```python
from build123d import *

# Parameters (mm, degrees)
F0_W      = 130
F0_H      = 75
F1_DEPTH  = 12
F3_DEPTH  = 319
F5_DEPTH  = 100
F6_W      = 220
F6_H      = 75
F7_DEPTH  = 12
F9_D      = 12
F9_DEPTH  = 12
F9_TIP    = 3.6051637142
F11_D     = 12
F11_DEPTH = 12
F11_TIP   = 3.6051637142


# Not quite as in the source:
# - a feature names something its author has since deleted; it is built from what else it names


with BuildPart() as f1:
    # F0 (on Top) → F1 (new body)
    with BuildSketch(Plane.XY):
        with Locations((65, -37.5)):
            Rectangle(F0_W, F0_H)
    extrude(amount=F1_DEPTH)

    # F2 (on face) → F3 (join)
    with BuildSketch(Plane.XY.offset(12)):
        with BuildLine():
            ThreePointArc((90.4, -18.45), (88.5401280605, -13.9598719395), (84.05, -12.1))
            Line((84.05, -12.1), (45.95, -12.1))
            ThreePointArc((45.95, -12.1), (41.4598719395, -13.9598719395), (39.6, -18.45))
            Line((39.6, -18.45), (39.6, -56.55))
            ThreePointArc((39.6, -56.55), (41.4598719395, -61.0401280605), (45.95, -62.9))
            Line((45.95, -62.9), (84.05, -62.9))
            ThreePointArc((84.05, -62.9), (88.5401280605, -61.0401280605), (90.4, -56.55))
            Line((90.4, -56.55), (90.4, -18.45))
        make_face()
        with BuildLine():
            Line((52.3, -18.45), (77.7, -18.45))
            ThreePointArc((77.7, -18.45), (82.1901280605, -20.3098719395), (84.05, -24.8))
            Line((84.05, -24.8), (84.05, -50.2))
            ThreePointArc((84.05, -50.2), (82.1901280605, -54.6901280605), (77.7, -56.55))
            Line((77.7, -56.55), (52.3, -56.55))
            ThreePointArc((52.3, -56.55), (47.8098719395, -54.6901280605), (45.95, -50.2))
            Line((45.95, -50.2), (45.95, -24.8))
            ThreePointArc((45.95, -24.8), (47.8098719395, -20.3098719395), (52.3, -18.45))
        make_face(mode=Mode.SUBTRACT)
    extrude(amount=F3_DEPTH)

    # F4 (on face) → F5 (cut)
    with BuildSketch(Plane.YZ.offset(90.4)):
        Polygon((-62.9, 305), (-12.1, 331), (-62.9, 331), align=None)
    extrude(amount=-F5_DEPTH, mode=Mode.SUBTRACT)

    # F6 (on face) → F7 (join)
    with BuildSketch(Plane(origin=(0, -136.7557973863, 267.1997887393), x_dir=(1, 0, 0), z_dir=(0, -0.4556049895, 0.8901820564))):
        with Locations((65, 111.5005595453)):
            Rectangle(F6_W, F6_H)
        with BuildLine():
            Line((90.4, 132.9006763674), (90.4, 90.1004427232))
            add(Edge.make_bspline(
                [(90.4, 90.1004427232), (90.4, 82.9670704491), (84.05, 82.9670704491)],
                knots=[4.7123889804, 4.7123889804, 4.7123889804, 6.2831853072, 6.2831853072, 6.2831853072], degree=2, weights=[1, 0.7071067812, 1]))
            Line((84.05, 82.9670704491), (45.95, 82.9670704491))
            add(Edge.make_bspline(
                [(45.95, 82.9670704491), (39.6, 82.9670704491), (39.6, 90.1004427232)],
                knots=[0, 0, 0, 1.5707963268, 1.5707963268, 1.5707963268], degree=2, weights=[1, 0.7071067812, 1]))
            Line((39.6, 90.1004427232), (39.6, 132.9006763674))
            add(Edge.make_bspline(
                [(39.6, 132.9006763674), (39.6, 140.0340486414), (45.95, 140.0340486414)],
                knots=[1.5707963268, 1.5707963268, 1.5707963268, 3.1415926536, 3.1415926536, 3.1415926536], degree=2, weights=[1, 0.7071067812, 1]))
            Line((45.95, 140.0340486414), (84.05, 140.0340486414))
            add(Edge.make_bspline(
                [(84.05, 140.0340486414), (90.4, 140.0340486414), (90.4, 132.9006763674)],
                knots=[3.1415926536, 3.1415926536, 3.1415926536, 4.7123889804, 4.7123889804, 4.7123889804], degree=2, weights=[1, 0.7071067812, 1]))
        make_face(mode=Mode.SUBTRACT)
        with BuildLine():
            add(Edge.make_bspline(
                [(90.4, 90.1004427232), (90.4, 82.9670704491), (84.05, 82.9670704491)],
                knots=[4.7123889804, 4.7123889804, 4.7123889804, 6.2831853072, 6.2831853072, 6.2831853072], degree=2, weights=[1, 0.7071067812, 1]))
            Line((90.4, 90.1004427232), (90.4, 132.9006763674))
            add(Edge.make_bspline(
                [(84.05, 140.0340486414), (90.4, 140.0340486414), (90.4, 132.9006763674)],
                knots=[3.1415926536, 3.1415926536, 3.1415926536, 4.7123889804, 4.7123889804, 4.7123889804], degree=2, weights=[1, 0.7071067812, 1]))
            Line((84.05, 140.0340486414), (45.95, 140.0340486414))
            add(Edge.make_bspline(
                [(39.6, 132.9006763674), (39.6, 140.0340486414), (45.95, 140.0340486414)],
                knots=[1.5707963268, 1.5707963268, 1.5707963268, 3.1415926536, 3.1415926536, 3.1415926536], degree=2, weights=[1, 0.7071067812, 1]))
            Line((39.6, 132.9006763674), (39.6, 90.1004427232))
            add(Edge.make_bspline(
                [(45.95, 82.9670704491), (39.6, 82.9670704491), (39.6, 90.1004427232)],
                knots=[0, 0, 0, 1.5707963268, 1.5707963268, 1.5707963268], degree=2, weights=[1, 0.7071067812, 1]))
            Line((45.95, 82.9670704491), (84.05, 82.9670704491))
        make_face()
        with BuildLine():
            Line((52.3, 132.9006763674), (77.7, 132.9006763674))
            add(Edge.make_bspline(
                [(77.7, 132.9006763674), (84.05, 132.9006763674), (84.05, 125.7673040934)],
                knots=[3.1415926536, 3.1415926536, 3.1415926536, 4.7123889804, 4.7123889804, 4.7123889804], degree=2, weights=[1, 0.7071067812, 1]))
            Line((84.05, 125.7673040934), (84.05, 97.2338149972))
            add(Edge.make_bspline(
                [(84.05, 97.2338149972), (84.05, 90.1004427232), (77.7, 90.1004427232)],
                knots=[4.7123889804, 4.7123889804, 4.7123889804, 6.2831853072, 6.2831853072, 6.2831853072], degree=2, weights=[1, 0.7071067812, 1]))
            Line((77.7, 90.1004427232), (52.3, 90.1004427232))
            add(Edge.make_bspline(
                [(52.3, 90.1004427232), (45.95, 90.1004427232), (45.95, 97.2338149972)],
                knots=[0, 0, 0, 1.5707963268, 1.5707963268, 1.5707963268], degree=2, weights=[1, 0.7071067812, 1]))
            Line((45.95, 97.2338149972), (45.95, 125.7673040934))
            add(Edge.make_bspline(
                [(45.95, 125.7673040934), (45.95, 132.9006763674), (52.3, 132.9006763674)],
                knots=[1.5707963268, 1.5707963268, 1.5707963268, 3.1415926536, 3.1415926536, 3.1415926536], degree=2, weights=[1, 0.7071067812, 1]))
        make_face(mode=Mode.SUBTRACT)
        with BuildLine():
            add(Edge.make_bspline(
                [(77.7, 132.9006763674), (84.05, 132.9006763674), (84.05, 125.7673040934)],
                knots=[3.1415926536, 3.1415926536, 3.1415926536, 4.7123889804, 4.7123889804, 4.7123889804], degree=2, weights=[1, 0.7071067812, 1]))
            Line((77.7, 132.9006763674), (52.3, 132.9006763674))
            add(Edge.make_bspline(
                [(45.95, 125.7673040934), (45.95, 132.9006763674), (52.3, 132.9006763674)],
                knots=[1.5707963268, 1.5707963268, 1.5707963268, 3.1415926536, 3.1415926536, 3.1415926536], degree=2, weights=[1, 0.7071067812, 1]))
            Line((45.95, 125.7673040934), (45.95, 97.2338149972))
            add(Edge.make_bspline(
                [(52.3, 90.1004427232), (45.95, 90.1004427232), (45.95, 97.2338149972)],
                knots=[0, 0, 0, 1.5707963268, 1.5707963268, 1.5707963268], degree=2, weights=[1, 0.7071067812, 1]))
            Line((52.3, 90.1004427232), (77.7, 90.1004427232))
            add(Edge.make_bspline(
                [(84.05, 97.2338149972), (84.05, 90.1004427232), (77.7, 90.1004427232)],
                knots=[4.7123889804, 4.7123889804, 4.7123889804, 6.2831853072, 6.2831853072, 6.2831853072], degree=2, weights=[1, 0.7071067812, 1]))
            Line((84.05, 97.2338149972), (84.05, 125.7673040934))
        make_face()
    extrude(amount=F7_DEPTH)

    # F9
    with Locations(Plane(origin=(0, -142.2230572602, 277.8819734162), x_dir=(1, 0, 0), z_dir=(0, -0.4556049895, 0.8901820564))):
        with Locations((-30, 89.0005595453), (100, 89.0005595453), (160, 89.0005595453), (160, 119.0005595453), (100, 119.0005595453), (30, 119.0005595453), (-30, 119.0005595453), (30, 89.0005595453)):
            Hole(F9_D / 2, depth=F9_DEPTH)
            with Locations((0, 0, -(F9_DEPTH + F9_TIP / 2))):  # 118° drill point
                Cone(0, F9_D / 2, F9_TIP, mode=Mode.SUBTRACT)

    # F11 (one way)
    with BuildSketch(Plane.XY.offset(12)):
        with Locations((15, -15), (15, -60), (115, -60), (115, -15)):
            Circle(F11_D / 2)
    extrude(amount=-F11_DEPTH, mode=Mode.SUBTRACT)
    with Locations(Plane.XY.offset(12)):
        with Locations((15, -15), (15, -60), (115, -60), (115, -15)):
            with Locations((0, 0, -(F11_DEPTH + F11_TIP / 2))):  # 118° drill point
                Cone(0, F11_D / 2, F11_TIP, mode=Mode.SUBTRACT)


solid = f1.part
```
Source: CAD feature listing. Evaluate the final solid. Frame: model axes, mm. A direction names the side the tool comes from. Give positions to 0.01 mm unless a question says otherwise; leave off trailing zeros. Write each loop counter-clockwise with the first axis right and the second up, starting at its lowest first coordinate (ties: lowest second). Pieces come first, ordered by that corner, then holes.
1. Pull-direction query (X, two-part tool) for faces 1 (the face through (84.05, -37, 166)), 2 (the face through (88.59, -14.01, 169.27)), 3 (the face through (93, -37, 12)); classes: +X half, -X half, draft (parallel to the pull), parting line (faces both ways), or undercut.
2. First-contact query: pin 1 (11.5 mm diameter, centred on x = 57, z = 125, fed in from +Y); pin 2 (12.5 mm diameter, centred on y = -36.5, z = 126.5, fed in from +X); pin 3 (2 mm diameter, centred on y = -34, z = 204, fed in from -X). Flat tips, straight axial feed; report the tip coordinate or a pass-through.
3. Access query for faces 4 (the face through (64.73, -37.23, 318.14)), 5 (the face through (65, -12.1, 169)), 6 (the face through (64, -37, 0)), 7 (the face through (63.46, -73.577, 306.181)), 8 (the face through (20.54, -62.3, 6.08)). Directions: +Z, -Z, +X, -X, +Y, -Y. A direction counts if a zero-diameter tool reaches every point of the face in a straight line with its end or side. Return the directions, or none.
4. Section query A-A (x = 15). Return the cut outline in (y, z).
5. Section query C-C (x = 59). Return the cut outline in (y, z).
6. Section query D-D (x = 115.5). Return the cut outline in (y, z), then the cut area to 3 significant figures.
7. Material intervals for line 1 along Y through (x, z) = (15, 6); line 2 along X through (y, z) = (-28, 307); line 3 along Z through (x, y) = (112, -39), sorted ascending.
8. Section query B-B (z = 151.5). Return the cut outline in (x, y), then the cut area to 3 significant figures.
Output values:
1. face 1: undercut
1. face 2: +X half
1. face 3: draft
2. pin 1: stops at y = -12.1
2. pin 2: stops at x = 90.4
2. pin 3: stops at x = 39.6
3. face 4: none
3. face 5: +X, -X, +Y
3. face 6: -Z, +X, -X, +Y, -Y
3. face 7: +X, -X, -Y
3. face 8: -Z
4. outline: (-76.35, 311.6) - (-70.88, 300.91) - (-4.12, 335.09) - (-9.59, 345.77) - close; (-75, 0) - (-66, 0) - (-66, 12) - (-75, 12) - close; (-54, 0) - (-21, 0) - (-21, 12) - (-54, 12) - close; (-9, 0) - (0, 0) - (0, 12) - (-9, 12) - close
5. outline: (-76.35, 311.6) - (-70.88, 300.91) - (-62.9, 305) - (-62.9, 12) - (-75, 12) - (-75, 0) - (0, 0) - (0, 12) - (-12.1, 12) - (-12.1, 331) - (-4.12, 335.09) - (-9.59, 345.77) - close; hole (-56.55, 12) - (-18.45, 12) - (-18.45, 327.75) - (-56.55, 308.25) - close
6. outline: (-76.35, 311.6) - (-70.88, 300.91) - (-4.12, 335.09) - (-9.59, 345.77) - close; (-75, 0) - (-65.98, 0) - (-65.98, 12) - (-75, 12) - close; (-54.02, 0) - (-20.98, 0) - (-20.98, 12) - (-54.02, 12) - close; (-9.02, 0) - (0, 0) - (0, 12) - (-9.02, 12) - close
6. area: 1,510 mm2
7. line 1: y = -75 to -66, -54 to -21, -9 to 0
7. line 2: x = 39.6 to 45.95, 84.05 to 90.4
7. line 3: z = 0 to 12, 317.23 to 330.71
8. outline: (39.6, -56.55) arc R6.35 ccw to (45.95, -62.9) - (84.05, -62.9) arc R6.35 ccw to (90.4, -56.55) - (90.4, -18.45) arc R6.35 ccw to (84.05, -12.1) - (45.95, -12.1) arc R6.35 ccw to (39.6, -18.45) - close; hole (45.95, -50.2) arc R6.35 ccw to (52.3, -56.55) - (77.7, -56.55) arc R6.35 ccw to (84.05, -50.2) - (84.05, -24.8) arc R6.35 ccw to (77.7, -18.45) - (52.3, -18.45) arc R6.35 ccw to (45.95, -24.8) - close
8. area: 1,130 mm2
